Check sheet for the modelled part. Datum: model origin and axes. Units: mm. Face numbers are marked on the shaded views. Round coordinates to 2 decimals unless told otherwise and drop trailing zeros. Write each loop counter-clockwise with the first axis right and the second up, starting at its lowest first coordinate (ties: lowest second). Pieces come first, ordered by that corner, then holes.
Item 1: Go/stop test with a flat-tipped pin: pin 1 Ø1 at (x, y) = (160.5, 126.5) entering from +Z. Record where the tip stops, or that it passes through.
Item 2: Cross-section at B-B on y = 85.5. Enter the section's corners in (x, z).
Item 3: Release check for a two-part mould opening along Y. For the marked faces 1 and 2 record: +Y half, -Y half, draft (parallel to the pull), parting line (faces both ways), or undercut.
Item 4: Cross-section at D-D on y = 131.5. Enter the section's corners in (x, z).
Item 5: Cross-section at C-C on x = 167. Enter the section's corners in (y, z).
Item 6: Material ranges on line 1 (Y direction, x = 58.5, z = 2.5); line 2 (X direction, y = 144, z = 1.1); line 3 (Y direction, x = 118, z = 1.15), recorded low to high.
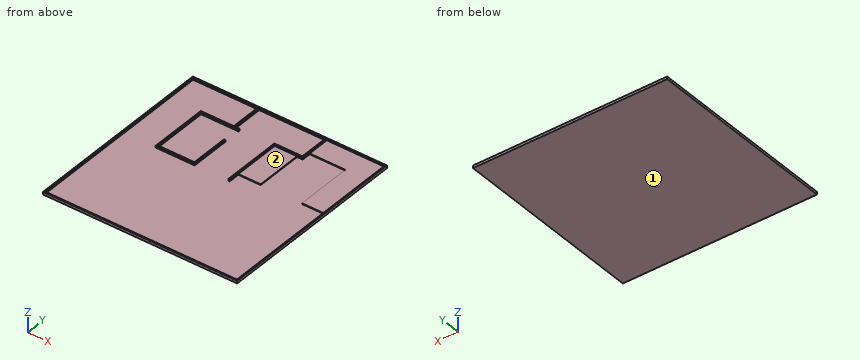
from build123d import *

# Parameters (mm, degrees)
F0_W     = 210
F0_H     = 210
F1_DEPTH = 0.8
F2_W     = 210
F2_H     = 210
F2_W_2   = 207.12
F2_H_2   = 207.12
F3_DEPTH = 2
F5_DEPTH = 2
F6_W     = 24.230769
F6_H     = 51.06
F7_DEPTH = 0.8


with BuildPart() as f1:
    # F0 (on Top) → F1 (new body)
    with BuildSketch(Plane.XY):
        with Locations((105, 105)):
            Rectangle(F0_W, F0_H)
    extrude(amount=F1_DEPTH)

    # F2 (on face) → F3 (join)
    with BuildSketch(Plane.XY.offset(0.8)):
        with Locations((105, 105)):
            Rectangle(F2_W, F2_H)
        with Locations((105, 105)):
            Rectangle(F2_W_2, F2_H_2, mode=Mode.SUBTRACT)
    extrude(amount=F3_DEPTH)

    # F4 (on face) → F5 (join, through all)
    with BuildSketch(Plane.XY.offset(0.8)):
        Polygon((145.963846, 174.812308), (145.963846, 208.56), (144.523846, 208.56), (144.523846, 176.252308), (114.235385, 176.252308), (114.235385, 111.636923), (115.675385, 111.636923), (115.675385, 174.812308), align=None)
        Polygon((72.889231, 174.812308), (72.889231, 208.56), (71.449231, 208.56), (71.449231, 174.812308), (35.766923, 174.812308), (35.766923, 111.636923), (77.889231, 111.636923), (77.889231, 154.598162), (76.449231, 154.598162), (76.449231, 113.076923), (37.206923, 113.076923), (37.206923, 173.372308), (77.889231, 173.372308), (77.889231, 174.812308), align=None)
    extrude(amount=F5_DEPTH)

    # F6 (on face) → F7 (join)
    with BuildSketch(Plane.XY.offset(0.8)):
        Polygon((208.56, 208.56), (145.963846, 208.56), (145.963846, 184.56), (184.56, 184.56), (184.56, 123.752308), (208.56, 123.752308), align=None)
        with Locations((127.790769, 149.282308)):
            Rectangle(F6_W, F6_H)
    extrude(amount=F7_DEPTH)


solid = f1.part
Response values:
1. pin 1: stops at z = 0.8
2. outline: (0, 0) - (210, 0) - (210, 2.8) - (208.56, 2.8) - (208.56, 0.8) - (1.44, 0.8) - (1.44, 2.8) - (0, 2.8) - close
3. face 1: draft
3. face 2: undercut
4. outline: (0, 0) - (210, 0) - (210, 2.8) - (208.56, 2.8) - (208.56, 1.6) - (184.56, 1.6) - (184.56, 0.8) - (139.91, 0.8) - (139.91, 1.6) - (115.68, 1.6) - (115.68, 2.8) - (114.24, 2.8) - (114.24, 0.8) - (77.89, 0.8) - (77.89, 2.8) - (76.45, 2.8) - (76.45, 0.8) - (37.21, 0.8) - (37.21, 2.8) - (35.77, 2.8) - (35.77, 0.8) - (1.44, 0.8) - (1.44, 2.8) - (0, 2.8) - close
5. outline: (0, 0) - (210, 0) - (210, 2.8) - (208.56, 2.8) - (208.56, 1.6) - (184.56, 1.6) - (184.56, 0.8) - (1.44, 0.8) - (1.44, 2.8) - (0, 2.8) - close
6. line 1: y = 0 to 1.44, 111.64 to 113.08, 173.37 to 174.81, 208.56 to 210
6. line 2: x = 0 to 1.44, 35.77 to 37.21, 76.45 to 77.89, 114.24 to 139.91, 184.56 to 210
6. line 3: y = 0 to 1.44, 123.75 to 176.25, 208.56 to 210
